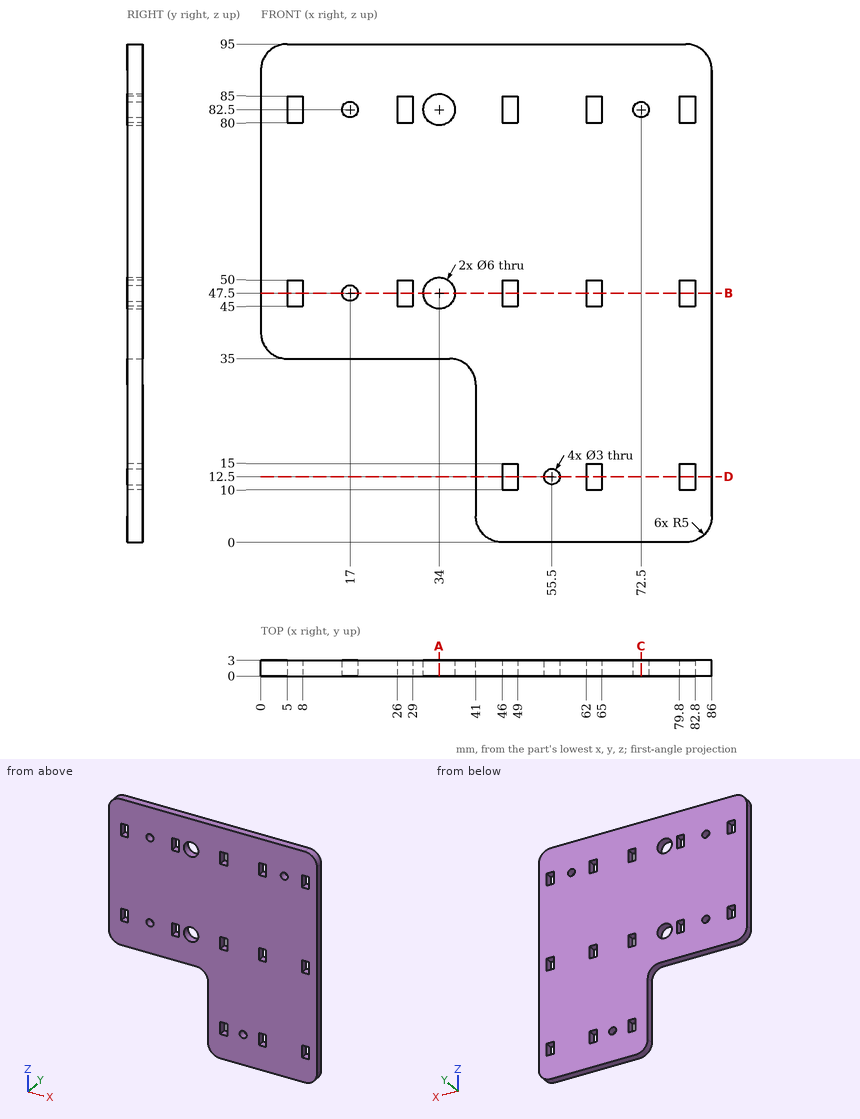
Could you check a few things on this drawing? It's one solid part, dimensions in mm from its lowest x, y, z. Give positions to 0.01 mm unless a question says otherwise; leave off trailing zeros. Order: outer loops, then holes, each group sorted by start corner. A loop starts at its lowest first (then second) coordinate and runs counter-clockwise, first axis right, second up. Notation, with made-up numbers: (-21.75, -22) - (-17.75, -22) arc R16 cw to (-17.75, -4) - close; hole circle Ø10 at (40, 86.25). An arc over 180 degrees is marked (long way). Answer as a JSON object with one key per item and string values. Group by question number.
Item 1: If we section it at C-C on x = 72.5: Please give me the cut outline in (y, z).
Item 2: For P1, Ø0.9, axis at x = 27, y = 1, coming from the -Z side, with a flat end and sliding along its axis, tell me the tip position at first contact or that it passes through.
Item 3: If we section it at D-D on z = 12.5: Please give me the cut outline in (x, y), and give its area (3 significant figures).
Item 4: Please list where these lines run through material, in increasing order: probe 1 along X at (y, z) = (1.55, 12.5); probe 2 along Z at (x, y) = (80, 1.2); probe 3 along Z at (x, y) = (34, 2).
Item 5: If we section it at B-B on z = 47.5: Give the number of separate pieces and of enclosed holes in the cut face, and give its area (3 significant figures).
Item 6: If we section it at A-A on x = 34: Please give me the cut outline in (y, z).
Result set:
{
 "1": {"outline": "(0, 0) - (3, 0) - (3, 81) - (0, 81) - close; (0, 84) - (3, 84) - (3, 95) - (0, 95) - close"},
 "2": {"P1": "z = 35"},
 "3": {"outline": "(41, 0) - (46, 0) - (46, 3) - (41, 3) - close; (49, 0) - (54, 0) - (54, 3) - (49, 3) - close; (57, 0) - (62, 0) - (62, 3) - (57, 3) - close; (65, 0) - (79.8, 0) - (79.8, 3) - (65, 3) - close; (82.8, 0) - (86, 0) - (86, 3) - (82.8, 3) - close", "area": "99.0 mm²"},
 "4": {"probe 1": "41 to 46, 49 to 54, 57 to 62, 65 to 79.8, 82.8 to 86", "probe 2": "0 to 10, 15 to 45, 50 to 80, 85 to 95", "probe 3": "35 to 44.5, 50.5 to 79.5, 85.5 to 95"},
 "5": {"separate pieces": "8", "enclosed holes": "0", "area": "186 mm²"},
 "6": {"outline": "(0, 35) - (3, 35) - (3, 44.5) - (0, 44.5) - close; (0, 50.5) - (3, 50.5) - (3, 79.5) - (0, 79.5) - close; (0, 85.5) - (3, 85.5) - (3, 95) - (0, 95) - close"}
}
